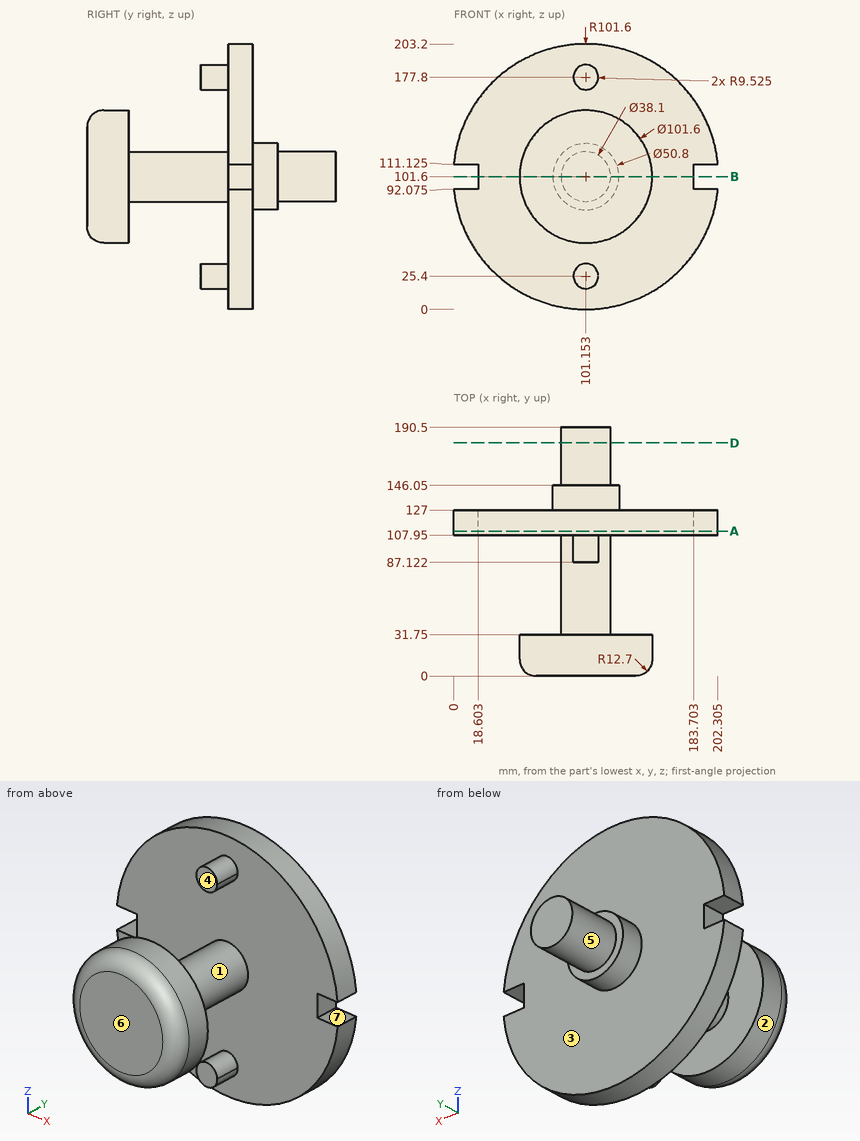
The figure shows three views and two pictorial views of one solid part (mm, origin at its lowest corner). Answer the questions. A direction names the side the tool comes from. Give positions to 0.01 mm unless a question says otherwise; leave off trailing zeros. Order: outer loops, then holes, each group sorted by start corner. A loop starts at its lowest first (then second) coordinate and runs counter-clockwise, first axis right, second up. Notation, with made-up numbers: (-31.75, -3.75) -> (25.25, -3.75) arc R30 ccw to (25.25, 23.25) -> close; hole circle Ø5 at (41.25, -39). An arc over 180 degrees is marked (long way). Answer as CSV lines item,"result". Start each with the question number.
(1) Section B-B, the plane z = 101.6 is taken. Write down the section's boundary in (x, y), plus the area to 3 significant figures.
(2) For a pull along Z with two mould halves and no side action, classify the marked faces 5, 6 and 7 as released by +Z, released by -Z, zero draft, split by the parting line, or undercut.
(3) Consider line 1 along Y through (x, z) = (93, 81.5); line 2 along Y through (x, z) = (36.5, 40); line 3 along Y through (x, z) = (99, 75). Determine where each line is inside the solid, lowest interval first.
(4) Each of these flat-tipped pins is pushed along its axis until it touches: pin 1 Ø15 at (x, y) = (194, 119) entering from +Z; pin 2 Ø4 at (x, z) = (140, 66) entering from +Y; pin 3 Ø20.5 at (x, y) = (190.5, 120.5) entering from -Z (1 decimal). Where does it stop, or does it pass through?
(5) Section A-A, the plane y = 111 is taken. Write down the section's boundary in (x, z) (1 decimal).
(6) Which of the six approach directions +Z, -Z, +X, -X, +Y, -Y give full straight-line access (tool end or side, diameter ignored) to the marked faces 1, 2, 3 and 4?
(7) Section D-D, the plane y = 178.5 is taken. Write down the section's boundary in (x, z), plus the area to 3 significant figures.
Entries:
1,outline,"(18.6, 107.95) -> (82.1, 107.95) -> (82.1, 31.75) -> (50.35, 31.75) -> (50.35, 12.7) arc R12.7 ccw to (63.05, 0) -> (139.25, 0) arc R12.7 ccw to (151.95, 12.7) -> (151.95, 31.75) -> (120.2, 31.75) -> (120.2, 107.95) -> (183.7, 107.95) -> (183.7, 127) -> (126.55, 127) -> (126.55, 146.05) -> (120.2, 146.05) -> (120.2, 190.5) -> (82.1, 190.5) -> (82.1, 146.05) -> (75.75, 146.05) -> (75.75, 127) -> (18.6, 127) -> close"
1,area,"11,900 mm²"
2,face 5,"split by the parting line"
2,face 6,"zero draft"
2,face 7,"undercut"
3,line 1,"0 to 31.75, 107.95 to 146.05"
3,line 2,"107.95 to 127"
3,line 3,"0 to 31.75, 107.95 to 127"
4,pin 1,"z = 156.72"
4,pin 2,"y = 127"
4,pin 3,"z = 37.8"
5,outline,"(0, 92.1) arc R101.6 ccw to (202.3, 92.1) -> (183.7, 92.1) -> (183.7, 111.1) -> (202.3, 111.1) arc R101.6 ccw to (0, 111.1) -> (18.6, 111.1) -> (18.6, 92.1) -> close"
6,face 1,"none"
6,face 2,"-Y"
6,face 3,"+Y"
6,face 4,"+Z, +X, -X, -Y"
7,outline,"circle Ø38.1 at (101.15, 101.6)"
7,area,"1,140 mm²"
